```python
from build123d import *

# Parameters (mm, degrees)
SKETCH1_W                = 13
SKETCH1_H                = 13
BOSS_EXTRUDE1_DEPTH      = 3.5
SKETCH2_W                = 22
SKETCH2_H                = 3.7
BOSS_EXTRUDE2_DEPTH      = 3.5
FILLET1_R                = 1.85
SKETCH3_R                = 0.5
CUT_EXTRUDE1_DEPTH       = 3.5
BOSS_EXTRUDE3_DEPTH      = 6.5
BOSS_EXTRUDE3_DEPTH_BACK = 3.5
SKETCH4_R                = 6.75
SKETCH5_R                = 0.5
CUT_EXTRUDE2_DEPTH       = 6.5
SKETCH6_R                = 6
CUT_EXTRUDE3_DEPTH       = 6.5


with BuildPart() as part:
    # Sketch1 → Boss-Extrude1 (new body)
    with BuildSketch(Plane.XY):
        Rectangle(SKETCH1_W, SKETCH1_H)
    extrude(amount=BOSS_EXTRUDE1_DEPTH)

    # Sketch2 → Boss-Extrude2 (add)
    with BuildSketch(Plane.XY.offset(3.5)):
        Rectangle(SKETCH2_W, SKETCH2_H)
    extrude(amount=-BOSS_EXTRUDE2_DEPTH)

    # Fillet1
    fillet1_edges = [part.edges().sort_by_distance(p)[0] for p in [
        (11, -1.85, 1.75),
        (11, 1.85, 1.75),
        (-11, -1.85, 1.75),
        (-11, 1.85, 1.75),
    ]]
    fillet(fillet1_edges, radius=FILLET1_R - 0.0001)  # a hair under: the kernel refuses the full size

    # Sketch3 → Cut-Extrude1 (cut)
    with BuildSketch(Plane.XY.offset(3.5)):
        with Locations((-9, 0)):
            Circle(SKETCH3_R)
        with Locations((9, 0)):
            Circle(SKETCH3_R)
    extrude(amount=-CUT_EXTRUDE1_DEPTH, mode=Mode.SUBTRACT)

    # Sketch4 → Boss-Extrude3 (add, two sides: drawn at the far end of the back side and taken through both)
    with BuildSketch(Plane.XY.offset(3.5).offset(-BOSS_EXTRUDE3_DEPTH_BACK)):
        Circle(SKETCH4_R)
    extrude(amount=BOSS_EXTRUDE3_DEPTH + BOSS_EXTRUDE3_DEPTH_BACK)

    # Sketch5 → Cut-Extrude2 (cut)
    with BuildSketch(Plane.XY.offset(10)):
        with Locations((0, 7)):
            Circle(SKETCH5_R)
        with Locations((1.324758711, 6.873500881)):
            Circle(SKETCH5_R)
        with Locations((2.60163719, 6.498575531)):
            Circle(SKETCH5_R)
        with Locations((3.784485722, 5.88877473)):
            Circle(SKETCH5_R)
        with Locations((4.83055308, 5.066138267)):
            Circle(SKETCH5_R)
        with Locations((5.702031664, 4.060398367)):
            Circle(SKETCH5_R)
        with Locations((6.367423967, 2.907905091)):
            Circle(SKETCH5_R)
        with Locations((6.802680978, 1.650312549)):
            Circle(SKETCH5_R)
        with Locations((6.992071374, 0.333073411)):
            Circle(SKETCH5_R)
        with Locations((6.928750093, -0.996203868)):
            Circle(SKETCH5_R)
        with Locations((6.615005731, -2.289475743)):
            Circle(SKETCH5_R)
        with Locations((6.062177826, -3.5)):
            Circle(SKETCH5_R)
        with Locations((5.29024702, -4.584025138)):
            Circle(SKETCH5_R)
        with Locations((4.327112904, -5.502371663)):
            Circle(SKETCH5_R)
        with Locations((3.207585652, -6.221848141)):
            Circle(SKETCH5_R)
        with Locations((1.972127898, -6.716450815)):
            Circle(SKETCH5_R)
        with Locations((0.665392303, -6.968303458)):
            Circle(SKETCH5_R)
        with Locations((-0.665392303, -6.968303458)):
            Circle(SKETCH5_R)
        with Locations((-1.972127898, -6.716450815)):
            Circle(SKETCH5_R)
        with Locations((-3.207585652, -6.221848141)):
            Circle(SKETCH5_R)
        with Locations((-4.327112904, -5.502371663)):
            Circle(SKETCH5_R)
        with Locations((-5.29024702, -4.584025138)):
            Circle(SKETCH5_R)
        with Locations((-6.062177826, -3.5)):
            Circle(SKETCH5_R)
        with Locations((-6.615005731, -2.289475743)):
            Circle(SKETCH5_R)
        with Locations((-6.928750093, -0.996203868)):
            Circle(SKETCH5_R)
        with Locations((-6.992071374, 0.333073411)):
            Circle(SKETCH5_R)
        with Locations((-6.802680978, 1.650312549)):
            Circle(SKETCH5_R)
        with Locations((-6.367423967, 2.907905091)):
            Circle(SKETCH5_R)
        with Locations((-5.702031664, 4.060398367)):
            Circle(SKETCH5_R)
        with Locations((-4.83055308, 5.066138267)):
            Circle(SKETCH5_R)
        with Locations((-3.784485722, 5.88877473)):
            Circle(SKETCH5_R)
        with Locations((-2.60163719, 6.498575531)):
            Circle(SKETCH5_R)
        with Locations((-1.324758711, 6.873500881)):
            Circle(SKETCH5_R)
    extrude(amount=-CUT_EXTRUDE2_DEPTH, mode=Mode.SUBTRACT)

    # Sketch6 → Cut-Extrude3 (cut)
    with BuildSketch(Plane.XY.offset(10)):
        Circle(SKETCH6_R)
    extrude(amount=-CUT_EXTRUDE3_DEPTH, mode=Mode.SUBTRACT)


solid = part.part
```
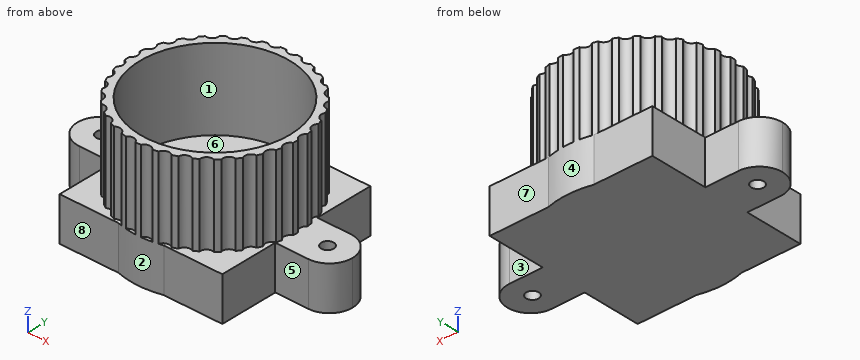
Input: part model. Units: mm. Frame: model coordinates. Face numbers are marked on the shaded views. A direction names the side the tool comes from. Round coordinates to 2 decimals unless told otherwise and drop trailing zeros. Loops run counter-clockwise (first coordinate to the right, second up) from the corner with the lowest first, then second, coordinate; pieces in that order, holes last. Notation, with made-up numbers: (62.25, 82) -> (80.25, 82) arc R19 ccw to (80.25, 91) -> close; hole circle Ø6 at (-1.5, -4.75). An arc over 180 degrees is marked (long way). One line per item, written item: value.
(1) Pin query (flat end, axial travel): pin 1 (1.8 mm diameter, centred on x = -3.5, z = 2, fed in from -Y); pin 2 (0.8 mm diameter, centred on x = 8, z = 2.5, fed in from +Y); pin 3 (1 mm diameter, centred on x = -4.5, z = 1.5, fed in from +Y). Return the tip coordinate at first contact, or that it passes through.
Geometry check:
pin 1: y = -6.5
pin 2: y = 1.85
pin 3: y = 6.5
(2) Material intervals for line 1 (Y direction, x = 9, z = 2.75); line 2 (X direction, y = -2.25, z = 7.25); line 3 (Z direction, x = -3.5, y = -6), sorted ascending. Write a range as [from, to].
Geometry check:
line 1: [-1.85, -0.5], [0.5, 1.85]
line 2: [-6.12, -5.56], [5.56, 6.12]
line 3: [0, 3.5]
(3) Section A-A (z = 1). Give the number of separate pieces and of enclosed holes in the cut face, plus the area to 3 significant figures.
Geometry check:
separate pieces: 1
enclosed holes: 2
area: 199 mm2
(4) Section C-C (y = -1). Return the cut outline in (x, z), plus the area to 3 significant figures.
Geometry check:
outline: (-10.71, 0) -> (10.71, 0) -> (10.71, 3.5) -> (6.43, 3.5) -> (6.43, 10) -> (5.92, 10) -> (5.92, 3.5) -> (-5.92, 3.5) -> (-5.92, 10) -> (-6.43, 10) -> (-6.43, 3.5) -> (-10.71, 3.5) -> close
area: 81.6 mm2
(5) Mould query, pull axis X, two halves, no side actions, for the marked faces 1, 2 and 3. Classes: pulls with the +X half, pulls with the -X half, needs draft (parallel to the pull), parting line crosses it, or undercut.
Geometry check:
face 1: undercut
face 2: parting line crosses it
face 3: needs draft
(6) Set-up query: the marked faces 4, 5, 6, 7 and 8. Return all of +Z, -Z, +X, -X, +Y, -Y with unobstructed straight access to the full face (end or side cutting, diameter ignored); none if empty.
Geometry check:
face 4: +Z, +Y
face 5: +Z, -Z, +X, -Y
face 6: +Z
face 7: +Z, -Z, +X, +Y
face 8: +Z, -Z, -X, -Y
(7) Section B-B (y = 1.5). Return the cut outline in (x, z), plus the area to 3 significant figures.
Geometry check:
outline: (-10.23, 0) -> (10.23, 0) -> (10.23, 3.5) -> (6.33, 3.5) -> (6.33, 10) -> (5.81, 10) -> (5.81, 3.5) -> (-5.81, 3.5) -> (-5.81, 10) -> (-6.33, 10) -> (-6.33, 3.5) -> (-10.23, 3.5) -> close
area: 78.3 mm2
